from build123d import *

# Parameters (mm, degrees)
SKETCH1_W           = 111.1
SKETCH1_H           = 51.3
BOSS_EXTRUDE1_DEPTH = 3
SKETCH2_W           = 111.1
SKETCH2_H           = 51.3
SKETCH2_W_2         = 105.3
SKETCH2_H_2         = 45.3
BOSS_EXTRUDE2_DEPTH = 40.5
SKETCH5_R           = 21
BOSS_EXTRUDE4_DEPTH = 15
SKETCH6_W           = 15.5
SKETCH6_H           = 37
CUT_EXTRUDE1_DEPTH  = 21
BOSS_EXTRUDE5_START = -1
SKETCH8_R           = 21
SKETCH8_W           = 12.3
SKETCH8_H           = 34.3
BOSS_EXTRUDE5_DEPTH = 1
BOSS_EXTRUDE6_START = -1
SKETCH9_R           = 21
SKETCH9_W           = 12.3
SKETCH9_H           = 34.3
BOSS_EXTRUDE6_DEPTH = 1
SKETCH10_W          = 126.244554882
SKETCH10_H          = 68.697179438
CUT_EXTRUDE3_DEPTH  = 53
SKETCH12_W          = 1
SKETCH12_H          = 1.5
BOSS_EXTRUDE8_DEPTH = 2
FILLET1_R           = 2
SKETCH13_R          = 3
CUT_EXTRUDE4_DEPTH  = 14


with BuildPart() as part:
    # Sketch1 → Boss-Extrude1 (new body)
    with BuildSketch(Plane(origin=(0, 0, 0), x_dir=(1, 0, 0), z_dir=(0, 1, 0))):
        Rectangle(SKETCH1_W, SKETCH1_H)
    extrude(amount=BOSS_EXTRUDE1_DEPTH)

    # Sketch2 → Boss-Extrude2 (add)
    with BuildSketch(Plane(origin=(0, 3, 0), x_dir=(1, 0, 0), z_dir=(0, 1, 0))):
        Rectangle(SKETCH2_W, SKETCH2_H)
        Rectangle(SKETCH2_W_2, SKETCH2_H_2, mode=Mode.SUBTRACT)
    extrude(amount=BOSS_EXTRUDE2_DEPTH)

    # Sketch5 → Boss-Extrude4 (add)
    with BuildSketch(Plane(origin=(0, 0, -25.65), x_dir=(-1, 0, 0), z_dir=(0, 0, -1))):
        with Locations((-27.775, 21.75)):
            Circle(SKETCH5_R)
        with Locations(Location((27.775, 21.75, 0), (0, 0, 180))):
            Circle(SKETCH5_R)
    extrude(amount=BOSS_EXTRUDE4_DEPTH)

    # Sketch6 → Cut-Extrude1 (cut)
    with BuildSketch(Plane(origin=(0, 0, -40.65), x_dir=(-1, 0, 0), z_dir=(0, 0, -1))):
        with Locations((-27.775, 21.75)):
            Rectangle(SKETCH6_W, SKETCH6_H)
        with Locations((27.775, 21.75)):
            Rectangle(SKETCH6_W, SKETCH6_H)
    extrude(amount=-CUT_EXTRUDE1_DEPTH, mode=Mode.SUBTRACT)

    # Sketch8 → Boss-Extrude5 (add)
    with BuildSketch(Plane(origin=(0, 0, -40.65), x_dir=(-1, 0, 0), z_dir=(0, 0, -1)).offset(BOSS_EXTRUDE5_START)):
        with Locations((-27.775, 21.75)):
            Circle(SKETCH8_R)
        with Locations((-27.775, 21.75)):
            Rectangle(SKETCH8_W, SKETCH8_H, mode=Mode.SUBTRACT)
    extrude(amount=BOSS_EXTRUDE5_DEPTH)

    # Sketch9 → Boss-Extrude6 (add)
    with BuildSketch(Plane(origin=(0, 0, -40.65), x_dir=(-1, 0, 0), z_dir=(0, 0, -1)).offset(BOSS_EXTRUDE6_START)):
        with Locations(Location((27.775, 21.75, 0), (0, 0, 180))):
            Circle(SKETCH9_R)
        with Locations((27.775, 21.75)):
            Rectangle(SKETCH9_W, SKETCH9_H, mode=Mode.SUBTRACT)
    extrude(amount=BOSS_EXTRUDE6_DEPTH)

    # Sketch10 → Cut-Extrude3 (cut)
    with BuildSketch(Plane.XY.offset(-22.65)):
        with Locations((0, 21.75)):
            Rectangle(SKETCH10_W, SKETCH10_H)
    extrude(amount=-CUT_EXTRUDE3_DEPTH, mode=Mode.SUBTRACT)

    # Sketch12 → Boss-Extrude8 (add)
    with BuildSketch(Plane(origin=(0, 0, -22.65), x_dir=(-1, 0, 0), z_dir=(0, 0, -1))):
        with Locations((52.15, 18.9)):
            Rectangle(SKETCH12_W, SKETCH12_H)
        with Locations((52.15, 7.95)):
            Rectangle(SKETCH12_W, SKETCH12_H)
        with Locations((-52.15, 18.9)):
            Rectangle(SKETCH12_W, SKETCH12_H)
        with Locations((-52.15, 24.6)):
            Rectangle(SKETCH12_W, SKETCH12_H)
        with Locations((52.15, 24.6)):
            Rectangle(SKETCH12_W, SKETCH12_H)
        with Locations((-52.15, 7.95)):
            Rectangle(SKETCH12_W, SKETCH12_H)
    extrude(amount=-BOSS_EXTRUDE8_DEPTH)

    # Fillet1
    fillet1_edges = [part.edges().sort_by_distance(p)[0] for p in [
        (55.55, 21.75, 25.65),
        (-55.55, 21.75, 25.65),
    ]]
    fillet(fillet1_edges, radius=FILLET1_R)

    # Sketch13 → Cut-Extrude4 (cut)
    with BuildSketch(Plane(origin=(-52.65, 0, 0), x_dir=(0, 0, -1), z_dir=(1, 0, 0))):
        with Locations((0, 21.75)):
            Circle(SKETCH13_R)
    extrude(amount=-CUT_EXTRUDE4_DEPTH, mode=Mode.SUBTRACT)


solid = part.part
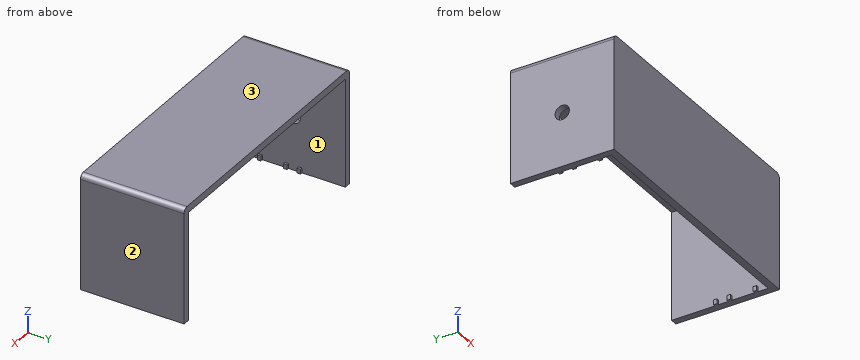
Could you check a few things on this model? Use its own coordinates, in mm. Face numbers are marked on the shaded views. Coordinates: 2 decimals unless noted, no trailing zeros. Write each loop counter-clockwise with the first axis right and the second up, starting at its lowest first coordinate (ties: lowest second). Pieces come first, ordered by that corner, then holes. Notation, with made-up numbers: M -31,80.25 L 14,80.25 A5 cw 14,89.25 Z; hole C 63.25,-8 d5. An arc over 180 degrees is marked long. One line per question, with ' | ' between items.
1) Imagine slicing it at A-A, the plane z = 0. Write out the boundary of the cut face in (x, y), and give its area (3 significant figures).
Checks:
outline: M -55.55,0 L 55.55,0 L 55.55,43.5 L 52.65,43.5 L 52.65,3 L -52.65,3 L -52.65,18.75 L -55.55,18.75 Z; M -55.55,24.75 L -52.65,24.75 L -52.65,43.5 L -55.55,43.5 Z | area: 551 mm²
2) For pin 1 Ø12 at (x, z) = (30.5, -4) entering from +Y; pin 2 Ø1.5 at (x, y) = (-8.5, 17.5) entering from -Z; pin 3 Ø0.5 at (x, z) = (-52, -22) entering from +Y, each with a flat end and sliding along its axis, tell me the tip position at first contact or that it passes through.
Checks:
pin 1: y = 3 | pin 2: z = 22.65 | pin 3: y = 25.35
3) Imagine slicing it at D-D, the plane y = 27.5. Write out the boundary of the cut face in (x, z).
Checks:
outline: M -55.55,-22.65 L -52.65,-22.65 L -52.65,22.65 L 52.65,22.65 L 52.65,-22.65 L 55.55,-22.65 L 55.55,23.65 A2 ccw 53.55,25.65 L -53.55,25.65 A2 ccw -55.55,23.65 Z
4) Imagine slicing it at C-C, the plane z = 11. Write out the boundary of the cut face in (x, y).
Checks:
outline: M -55.55,0 L 55.55,0 L 55.55,43.5 L 52.65,43.5 L 52.65,3 L -52.65,3 L -52.65,43.5 L -55.55,43.5 Z
5) I need wall thicknesses on probe 1 along X at (y, z) = (25, 12); probe 2 along Y at (x, z) = (-53, 0); probe 3 along Z at (x, y) = (6, 19.5). Which ranges of each line are inside material? Lowest first, please. Write a range as [from, to].
Checks:
probe 1: [-55.55, -52.65], [52.65, 55.55] | probe 2: [0, 18.75], [24.75, 43.5] | probe 3: [22.65, 25.65]
6) Imagine slicing it at B-B, the plane y = 21.75. Write out the boundary of the cut face in (x, z), and give its area (3 significant figures).
Checks:
outline: M -55.55,-22.65 L -52.65,-22.65 L -52.65,-3 L -55.55,-3 Z; M -55.55,3 L -52.65,3 L -52.65,22.65 L 52.65,22.65 L 52.65,-22.65 L 55.55,-22.65 L 55.55,23.65 A2 ccw 53.55,25.65 L -53.55,25.65 A2 ccw -55.55,23.65 Z | area: 577 mm²
7) If we mould it in two halves opening along X, with no side actions, what happens to the marked faces 1, 2 and 3? For each: released by +X, released by -X, zero draft, split by the parting line, or undercut.
Checks:
face 1: undercut | face 2: released by +X | face 3: zero draft
